from build123d import *

# Parameters (mm, degrees)
SKETCH_1_R                  = 31
SKETCH_1_R_2                = 2.25
SKETCH_1_R_3                = 1.35
EXTRUDE_1_DEPTH             = 3
EXTRUDE_START               = -3
EXTRUDE_2_DEPTH             = 3
SKETCH_7_R                  = 15
CUT_EXTRUDE_1_DEPTH         = 3
SM_EDGE_FLANGE_1_DEPTH      = 20
SM_EDGE_FLANGE_1_BEND_DEPTH = 20
SKETCH_14_R                 = 2.1
CUT_EXTRUDE_2_DEPTH         = 119.156675647
FILLET_1_R                  = 3


# Sheet-metal steps are written as plain solids
with BuildPart() as part:
    # Sketch 1 → 凸台-拉伸1 (new body)
    with BuildSketch(Plane.XY):
        Circle(SKETCH_1_R)
        with Locations((0, 27)):
            Circle(SKETCH_1_R_2, mode=Mode.SUBTRACT)
        with Locations((0, -27)):
            Circle(SKETCH_1_R_3, mode=Mode.SUBTRACT)
        with Locations((23.382685902, -13.5)):
            Circle(SKETCH_1_R_2, mode=Mode.SUBTRACT)
        with Locations((-23.382685902, 13.5)):
            Circle(SKETCH_1_R_3, mode=Mode.SUBTRACT)
        with Locations((-23.382685902, -13.5)):
            Circle(SKETCH_1_R_2, mode=Mode.SUBTRACT)
        with Locations((23.382685902, 13.5)):
            Circle(SKETCH_1_R_3, mode=Mode.SUBTRACT)
    extrude(amount=EXTRUDE_1_DEPTH)

    # Sketch 2 → 凸台-拉伸2 (add)
    with BuildSketch(Plane.XY.offset(3).offset(EXTRUDE_START)):
        with BuildLine():
            ThreePointArc((-10.236969115, -29.260971674), (-30.820342362, -3.332641094), (-16.255261315, 26.396334586))
            Line((-16.255261315, 26.396334586), (-51, 5))
            Line((-51, 5), (-51, -15))
            Line((-51, -15), (-10.236969115, -29.260971674))
        make_face()
        with BuildLine():
            Line((51, -15), (51, 5))
            Line((51, 5), (16.255261315, 26.396334586))
            ThreePointArc((16.255261315, 26.396334586), (27.063934496, 15.117653575), (31, 0))
            ThreePointArc((31, 0), (25.281871396, -17.939536747), (10.236969115, -29.260971674))
            Line((10.236969115, -29.260971674), (51, -15))
        make_face()
    extrude(amount=EXTRUDE_2_DEPTH)

    # 草图7 → 切除-拉伸1 (cut)
    with BuildSketch(Plane.XY.offset(3)):
        Circle(SKETCH_7_R)
    extrude(amount=-CUT_EXTRUDE_1_DEPTH, mode=Mode.SUBTRACT)

    # 边线-法兰1 section (across the edge) → 边线-法兰1 (add)
    with BuildSketch(Plane(origin=(-52, 5, 3), x_dir=(1, 0, 0), z_dir=(0, -1, 0))):
        with BuildLine():
            Line((-3, 1), (-3, 27))
            Line((-3, 27), (0, 27))
            Line((0, 27), (0, 1))
            ThreePointArc((0, 1), (0.292893219, 0.292893219), (1, 0))
            Line((1, 0), (1, -3))
            ThreePointArc((1, -3), (-1.828427125, -1.828427125), (-3, 1))
        make_face()
    extrude(amount=SM_EDGE_FLANGE_1_DEPTH)

    # 边线-法兰1 section 2 (across the edge) → 边线-法兰1 bend (add)
    with BuildSketch(Plane(origin=(52, -15, 3), x_dir=(-1, 0, 0), z_dir=(0, 1, 0))):
        with BuildLine():
            Line((-3, 1), (-3, 27))
            Line((-3, 27), (0, 27))
            Line((0, 27), (0, 1))
            ThreePointArc((0, 1), (0.292893219, 0.292893219), (1, 0))
            Line((1, 0), (1, -3))
            ThreePointArc((1, -3), (-1.828427125, -1.828427125), (-3, 1))
        make_face()
    extrude(amount=SM_EDGE_FLANGE_1_BEND_DEPTH)

    # 草图14 → 切除-拉伸2 (cut, through all)
    with BuildSketch(Plane(origin=(55, 0, 0), x_dir=(0, 0, -1), z_dir=(1, 0, 0))):
        with Locations((-16, -5)):
            Circle(SKETCH_14_R)
        with Locations((-26, -5)):
            Circle(SKETCH_14_R)
    extrude(amount=-CUT_EXTRUDE_2_DEPTH, mode=Mode.SUBTRACT)

    # 圆角1
    fillet_1_edges = [part.edges().sort_by_distance(p)[0] for p in [
        (-53.5, 5, 30),
        (-53.5, -15, 30),
        (53.5, -15, 30),
        (53.5, 5, 30),
    ]]
    fillet(fillet_1_edges, radius=FILLET_1_R)


solid = part.part
Design review of the part built by this model. Coordinates are the model's own, in mm. A direction names the side the tool comes from. Round coordinates to 2 decimals unless told otherwise and drop trailing zeros. Write each loop counter-clockwise with the first axis right and the second up, starting at its lowest first coordinate (ties: lowest second). Pieces come first, ordered by that corner, then holes. Notation, with made-up numbers: (68, 51) - (83, 51) arc R21 cw to (83, 75) - close; hole circle Ø1 at (26, -36). An arc over 180 degrees is marked (long way). Return JSON: item names as keys, results as strings. Group by question number.
Item 1: Machinability: for faces 1 (the face through (11, -13, 3)), 2 (the face through (54, -5, 30)), which of the approach directions +Z, -Z, +X, -X, +Y, -Y give a long, thin tool a straight path to every point of the face, cutting with its end or side? Answer none if there is none.
Item 2: We need section B-B on y = -27. Write out the cut boundary in (x, z), and give its area (3 significant figures).
Item 3: For probe 1 along Y at (x, z) = (-53.4, 16); probe 2 along X at (y, z) = (-14, 17); probe 3 along Z at (x, y) = (6, -16), list the stretches that pass through material, from the lowest coordinate up. Write a range as [from, to].
Item 4: We need section A-A on z = 16. Write out the cut boundary in (x, y).
Item 5: The part is to be moulded in two halves that separate along Y. For faces 3 (the face through (-0.29, -28.32, 1.48)), 4 (the face through (53.797, -5.14, 1.141)), 5 (the face through (53.52, -7.05, 16.46)), 6 (the face through (33.87, 15.55, 1.48)), say which applies: pulls with the +Y half, pulls with the -Y half, needs draft (parallel to the pull), parting line crosses it, or undercut.
Item 6: Insertion check: P1, Ø4.5, axis at x = 53, z = 19, coming from the -Y side; P2, Ø1, axis at x = 16.5, y = 18, coming from the +Z side; P3, Ø1.2, axis at x = -53, z = 14, coming from the +Y side. Each pin has a flat end and moves straight along its axis. Give the tip position at first contact, or say it passes through.
Item 7: We need section D-D on y = 0. Write out the cut boundary in (x, z), and give its area (3 significant figures).
Item 8: We need section C-C on x = -12.5. Write out the cut boundary in (y, z), and give its area (3 significant figures).
Model answer:
{
 "1": {"face 1": "+Z, +Y, -Y", "face 2": "+Z, +X, -X, +Y, -Y"},
 "2": {"outline": "(-16.7, 0) - (-1.35, 0) - (-1.35, 3) - (-16.7, 3) - close; (1.35, 0) - (16.7, 0) - (16.7, 3) - (1.35, 3) - close", "area": "92.1 mm²"},
 "3": {"probe 1": "y = [-15, -7.1], [-2.9, 5]", "probe 2": "x = [-55, -52], [52, 55]", "probe 3": "z = [0, 3]"},
 "4": {"outline": "(-55, -15) - (-52, -15) - (-52, -7.1) - (-55, -7.1) - close; (-55, -2.9) - (-52, -2.9) - (-52, 5) - (-55, 5) - close; (52, -15) - (55, -15) - (55, -7.1) - (52, -7.1) - close; (52, -2.9) - (55, -2.9) - (55, 5) - (52, 5) - close"},
 "5": {"face 3": "undercut", "face 4": "needs draft", "face 5": "undercut", "face 6": "pulls with the +Y half"},
 "6": {"P1": "stops at y = -15", "P2": "stops at z = 3", "P3": "stops at y = 5"},
 "7": {"outline": "(-55, 4) arc R4 ccw to (-51, 0) - (-15, 0) - (-15, 3) - (-51, 3) arc R1 cw to (-52, 4) - (-52, 30) - (-55, 30) - close; (15, 0) - (51, 0) arc R4 ccw to (55, 4) - (55, 30) - (52, 30) - (52, 4) arc R1 cw to (51, 3) - (15, 3) - close", "area": "396 mm²"},
 "8": {"outline": "(-28.47, 0) - (-8.29, 0) - (-8.29, 3) - (-28.47, 3) - close; (8.29, 0) - (28.37, 0) - (28.37, 3) - (8.29, 3) - close", "area": "121 mm²"}
}
